Geometry check sheet. Reference: the model listing, model coordinates, mm. Face numbers are marked on the shaded views. A direction names the side the tool comes from. Coordinates: 2 decimals unless noted, no trailing zeros. Write each loop counter-clockwise with the first axis right and the second up, starting at its lowest first coordinate (ties: lowest second). Pieces come first, ordered by that corner, then holes.
from build123d import *

# Parameters (mm, degrees)
F0_R     = 5
F1_DEPTH = 15
F3_DEPTH = 6
F5_DEPTH = 6


with BuildPart() as f1:
    # F0 (on Front) → F1 (new body)
    with BuildSketch(Plane.XZ):
        Circle(F0_R)
    extrude(amount=F1_DEPTH)

    # F2 (on face) → F3 (cut)
    with BuildSketch(Plane.XZ.offset(15)):
        with BuildLine():
            ThreePointArc((4, 3), (0, 5), (-4, 3))
            Line((-4, 3), (4, 3))
        make_face()
    extrude(amount=-F3_DEPTH, mode=Mode.SUBTRACT)

    # F4 (on face) → F5 (cut)
    with BuildSketch(Plane(origin=(0, 0, 0), x_dir=(-1, 0, 0), z_dir=(0, 1, 0))):
        with BuildLine():
            ThreePointArc((4, 3), (0, 5), (-4, 3))
            Line((-4, 3), (4, 3))
        make_face()
    extrude(amount=-F5_DEPTH, mode=Mode.SUBTRACT)


solid = f1.part
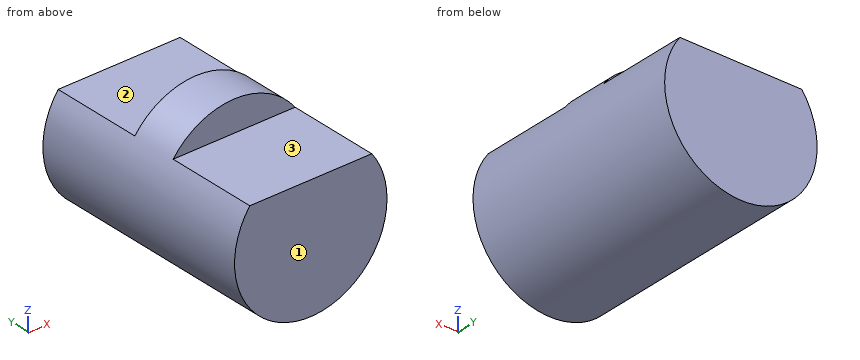
1. Thickness scan on line 1 along Y through (x, z) = (3.5, 3.5); line 2 along Z through (x, y) = (-0.75, -7.5); line 3 along X through (y, z) = (-6, -1.75). Record the ranges inside material, lowest first.
Computed values:
line 1: y = -9 to -6
line 2: z = -4.94 to 4.94
line 3: x = -4.68 to 4.68
2. Gauge pin test, flat ends, axial feed: pin 1 Ø6 at (y, z) = (-5, -3.5) entering from -X; pin 2 Ø2 at (x, y) = (-1.5, -10) entering from -Z; pin 3 Ø1 at (x, z) = (-1.5, 4.5) entering from +Y. Record the tip position at first contact, or that the pin passes through.
Computed values:
pin 1: stops at x = -4.97
pin 2: stops at z = -4.97
pin 3: stops at y = -6
3. Sectioned sample at B-B, the plane y = -6.5. Record the boundary of the cut face in (x, z).
Computed values:
outline: circle Ø10 at (0, 0)
4. Access from +Z, -Z, +X, -X, +Y, -Y to the whole of each face (thin tool, end or side, straight path). Record for the marked faces 1, 2 and 3.
Computed values:
face 1: +Z, -Z, +X, -X, -Y
face 2: +Z, +X, -X, +Y
face 3: +Z, +X, -X, -Y
5. Sectioned sample at C-C, the plane z = -1.5. Record the boundary of the cut face in (x, y), and give its area (3 significant figures).
Computed values:
outline: (-4.77, -15) - (4.77, -15) - (4.77, 0) - (-4.77, 0) - close
area: 143 mm2
6. Sectioned sample at D-D, the plane x = 2. Record the boundary of the cut face in (y, z).
Computed values:
outline: (-15, -4.58) - (0, -4.58) - (0, 3) - (-6, 3) - (-6, 4.58) - (-9, 4.58) - (-9, 3) - (-15, 3) - close
7. Sectioned sample at A-A, the plane x = 0. Record the boundary of the cut face in (y, z), and give its area (3 significant figures).
Computed values:
outline: (-15, -5) - (0, -5) - (0, 3) - (-6, 3) - (-6, 5) - (-9, 5) - (-9, 3) - (-15, 3) - close
area: 126 mm2
